Input: part model. Units: mm. Frame: model coordinates. Face numbers are marked on the shaded views. A direction names the side the tool comes from. Give positions to 0.01 mm unless a question says otherwise; leave off trailing zeros. Loops run counter-clockwise (first coordinate to the right, second up) from the corner with the lowest first, then second, coordinate; pieces in that order, holes last. Notation, with made-up numbers: M 31.25,14.25 L 56.25,14.25 A24 ccw 56.25,30.25 Z; hole C 75,46.25 d6. An arc over 180 degrees is marked long. Return JSON: item names as keys, results as strings. Group by question number.
```python
from build123d import *

# Parameters (mm, degrees)
EXTRUDE_1_DEPTH                 = 30
SKETCH_2_W                      = 3
SKETCH_2_H                      = 3
EXTRUDE_2_DEPTH                 = 1
EXTRUDE_START                   = -4
EXTRUDE_3_DEPTH                 = 5
CUT_EXTRUDE_1_REACH             = 52.312
CUT_EXTRUDE_1_DIRECTION_2_REACH = 52.312
FILLET_1_R                      = 0.1
PATTERN_LINEAR_1_COUNT          = 2
PATTERN_LINEAR_1_PITCH          = 15
PATTERN_LINEAR_1_COUNT_DIR2     = 2
PATTERN_LINEAR_1_PITCH_DIR2     = 15
FILLET_1_OF_PATTERN_LINEAR_1_R  = 0.1
FILLET_2_R                      = 0.2


with BuildPart() as part:
    # Sketch 1 → Extrude 1 (new body)
    with BuildSketch(Plane.XY):
        Polygon((-25.328427125, 0), (25.328427125, 0), (37.5, 12.171572875), (37.5, 15), (23.98, 2), (-23.98, 2), (-37.5, 15), (-37.5, 12.171572875), align=None)
    extrude(amount=-EXTRUDE_1_DEPTH)

    # Sketch 2 → Extrude 2 (add)
    with BuildSketch(Plane(origin=(0, 2, 0), x_dir=(1, 0, 0), z_dir=(0, 1, 0))):
        with Locations((0, 7.5)):
            Rectangle(SKETCH_2_W, SKETCH_2_H)
    extrude_2 = extrude(amount=EXTRUDE_2_DEPTH)

    # Sketch 3 → Extrude 3 (add)
    with BuildSketch(Plane.XY.offset(-6).offset(EXTRUDE_START)):
        with BuildLine():
            Line((-1.95, 4.5), (1.95, 4.5))
            Line((1.95, 4.5), (1.95, 3.555590279))
            ThreePointArc((1.95, 3.555590279), (1.780042303, 3.088161527), (1.5, 2.677124344))
            Line((1.5, 2.677124344), (-1.5, 2.677124344))
            ThreePointArc((-1.5, 2.677124344), (-1.780042303, 3.088161527), (-1.95, 3.555590279))
            Line((-1.95, 3.555590279), (-1.95, 4.5))
        make_face()
    extrude_3 = extrude(amount=EXTRUDE_3_DEPTH)

    # Sketch 4 → Cut-Extrude 1 (cut, up to next)
    with BuildSketch(Plane(origin=(0, 0, 0), x_dir=(0, 0, -1), z_dir=(1, 0, 0)), mode=Mode.PRIVATE) as cut_extrude_1_sk1:
        with BuildLine():
            Line((10, 4.5), (9.45, 4.5))
            Line((9.45, 4.5), (9.45, 3.555590279))
            ThreePointArc((9.45, 3.555590279), (9.280042303, 3.088161527), (9, 2.677124344))
            Line((9, 2.677124344), (10, 2.677124344))
            Line((10, 2.677124344), (10, 4.5))
        make_face()
    cut_extrude_1_tool1 = extrude(cut_extrude_1_sk1.sketch, amount=-CUT_EXTRUDE_1_REACH, mode=Mode.PRIVATE) & part.part
    # Sketch 4 → Cut-Extrude 1 (cut, up to next)
    with BuildSketch(Plane(origin=(0, 0, 0), x_dir=(0, 0, -1), z_dir=(1, 0, 0)), mode=Mode.PRIVATE) as cut_extrude_1_sk2:
        with BuildLine():
            Line((5, 4.5), (5, 2.677124344))
            Line((5, 2.677124344), (6, 2.677124344))
            ThreePointArc((6, 2.677124344), (5.719957697, 3.088161527), (5.55, 3.555590279))
            Line((5.55, 3.555590279), (5.55, 4.5))
            Line((5.55, 4.5), (5, 4.5))
        make_face()
    cut_extrude_1_tool2 = extrude(cut_extrude_1_sk2.sketch, amount=-CUT_EXTRUDE_1_REACH, mode=Mode.PRIVATE) & part.part
    cut_extrude_1_1 = cut_extrude_1_tool1.solids().sort_by_distance((0, 3.500125, -9.669375))[0]
    add(cut_extrude_1_1, mode=Mode.SUBTRACT)
    cut_extrude_1_2 = cut_extrude_1_tool2.solids().sort_by_distance((0, 3.500125, -5.330625))[0]
    add(cut_extrude_1_2, mode=Mode.SUBTRACT)
    cut_extrude_1 = cut_extrude_1_1 + cut_extrude_1_2  # Cut-Extrude 1 as one shape, for the pattern or mirror that repeats it

    # Sketch 4 → Cut-Extrude 1 direction 2 (cut, up to next)
    with BuildSketch(Plane(origin=(0, 0, 0), x_dir=(0, 0, -1), z_dir=(1, 0, 0)), mode=Mode.PRIVATE) as cut_extrude_1_direction_2_sk1:
        with BuildLine():
            Line((10, 4.5), (9.45, 4.5))
            Line((9.45, 4.5), (9.45, 3.555590279))
            ThreePointArc((9.45, 3.555590279), (9.280042303, 3.088161527), (9, 2.677124344))
            Line((9, 2.677124344), (10, 2.677124344))
            Line((10, 2.677124344), (10, 4.5))
        make_face()
    cut_extrude_1_direction_2_tool1 = extrude(cut_extrude_1_direction_2_sk1.sketch, amount=CUT_EXTRUDE_1_DIRECTION_2_REACH, mode=Mode.PRIVATE) & part.part
    # Sketch 4 → Cut-Extrude 1 direction 2 (cut, up to next)
    with BuildSketch(Plane(origin=(0, 0, 0), x_dir=(0, 0, -1), z_dir=(1, 0, 0)), mode=Mode.PRIVATE) as cut_extrude_1_direction_2_sk2:
        with BuildLine():
            Line((5, 4.5), (5, 2.677124344))
            Line((5, 2.677124344), (6, 2.677124344))
            ThreePointArc((6, 2.677124344), (5.719957697, 3.088161527), (5.55, 3.555590279))
            Line((5.55, 3.555590279), (5.55, 4.5))
            Line((5.55, 4.5), (5, 4.5))
        make_face()
    cut_extrude_1_direction_2_tool2 = extrude(cut_extrude_1_direction_2_sk2.sketch, amount=CUT_EXTRUDE_1_DIRECTION_2_REACH, mode=Mode.PRIVATE) & part.part
    cut_extrude_1_direction_2_1 = cut_extrude_1_direction_2_tool1.solids().sort_by_distance((0, 3.500125, -9.669375))[0]
    add(cut_extrude_1_direction_2_1, mode=Mode.SUBTRACT)
    cut_extrude_1_direction_2_2 = cut_extrude_1_direction_2_tool2.solids().sort_by_distance((0, 3.500125, -5.330625))[0]
    add(cut_extrude_1_direction_2_2, mode=Mode.SUBTRACT)
    cut_extrude_1_direction_2 = cut_extrude_1_direction_2_1 + cut_extrude_1_direction_2_2  # Cut-Extrude 1 direction 2 as one shape, for the pattern or mirror that repeats it

    # Fillet 1
    fillet_1_edges = [part.edges().sort_by_distance(p)[0] for p in [
        (1.95, 4.5, -7.5),
        (-1.95, 4.5, -7.5),
        (0, 4.5, -9.45),
        (0, 4.5, -5.55),
    ]]
    fillet(fillet_1_edges, radius=FILLET_1_R)

    # Pattern Linear 1: Extrude 2, Extrude 3, Cut-Extrude 1, Cut-Extrude 1 direction 2 2 × 2
    with Locations(*[Vector(1, 0, 0) * (i * PATTERN_LINEAR_1_PITCH) + Vector(-1, 0, 0) * (j * PATTERN_LINEAR_1_PITCH_DIR2) for i in range(PATTERN_LINEAR_1_COUNT) for j in range(PATTERN_LINEAR_1_COUNT_DIR2) if (i, j) != (0, 0)]):
        add(extrude_2)
        add(extrude_3)
        add(cut_extrude_1, mode=Mode.SUBTRACT)
        add(cut_extrude_1_direction_2, mode=Mode.SUBTRACT)

    # Fillet 1 of Pattern Linear 1
    fillet_1_of_pattern_linear_1_edges = [part.edges().sort_by_distance(p)[0] for p in [
        (-13.05, 4.5, -7.5),
        (-16.95, 4.5, -7.5),
        (-15, 4.5, -9.45),
        (-15, 4.5, -5.55),
        (16.95, 4.5, -7.5),
        (13.05, 4.5, -7.5),
        (15, 4.5, -9.45),
        (15, 4.5, -5.55),
        (1.95, 4.5, -7.5),
        (-1.95, 4.5, -7.5),
        (0, 4.5, -9.45),
        (0, 4.5, -5.55),
    ]]
    fillet(fillet_1_of_pattern_linear_1_edges, radius=FILLET_1_OF_PATTERN_LINEAR_1_R)

    # Fillet 2
    fillet_2_edges = [part.edges().sort_by_distance(p)[0] for p in [
        (0, 0, -30),
        (-31.414213562, 6.085786438, 0),
        (-37.5, 13.585786438, 0),
        (31.414213562, 6.085786438, -30),
        (-37.5, 15, -15),
        (37.5, 15, -15),
        (25.328427125, 0, -15),
        (-25.328427125, 0, -15),
        (37.5, 13.585786438, -30),
        (30.74, 8.5, -30),
        (0, 2, -30),
        (-30.74, 8.5, -30),
        (-37.5, 13.585786438, -30),
        (-31.414213562, 6.085786438, -30),
        (-30.74, 8.5, 0),
        (0, 2, 0),
        (30.74, 8.5, 0),
        (37.5, 13.585786438, 0),
        (31.414213562, 6.085786438, 0),
        (0, 0, 0),
    ]]
    fillet(fillet_2_edges, radius=FILLET_2_R)


solid = part.part
```
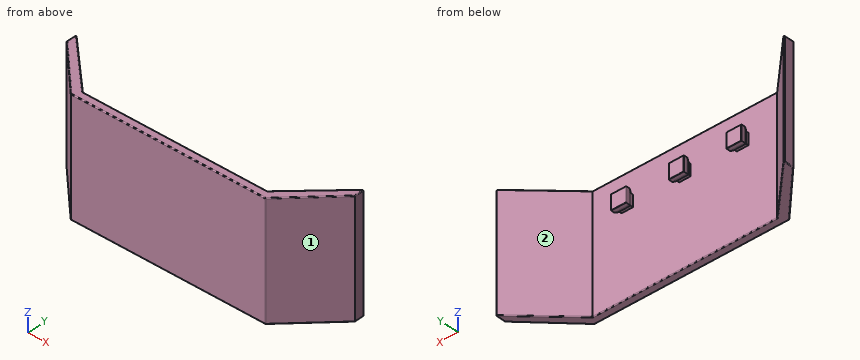
Item 1: Section B-B, the plane x = 4.5. Return loops of the section in (y, z), then the cut area to 3 significant figures.
Item 2: Section A-A, the plane z = -3.25. Return loops of the section in (x, y).
Item 3: First-contact query: pin 1 Ø0.7 at (y, z) = (4, -8) entering from -X; pin 2 Ø10 at (x, z) = (-24.5, -22.5) entering from +Y; pin 3 Ø0.5 at (y, z) = (2, -7) entering from +X. Flat tips, straight axial feed; report the tip coordinate or a pass-through.
Item 4: Reachability of the marked faces 1 and 2 from +Z, -Z, +X, -X, +Y, -Y: full face, straight path, thin tool, end or side. Return the list, or none.
Item 5: Material intervals for line 1 (X direction, y = 8.5, z = -21.75); line 2 (X direction, y = 11.5, z = -25.75); line 3 (Y direction, x = 11.5, z = -13.25), sorted ascending. Write a range as from..to.
Answer below:
{
 "1": {"outline": "M 0,-29.8 A0.2 ccw 0.2,-30 L 1.8,-30 A0.2 ccw 2,-29.8 L 2,-0.2 A0.2 ccw 1.8,0 L 0.2,0 A0.2 ccw 0,-0.2 Z", "area": "60.0 mm^2"},
 "2": {"outline": "M -37.5,12.17 L -25.39,0.06 A0.2 ccw -25.25,0 L 25.25,0 A0.2 ccw 25.39,0.06 L 37.5,12.17 L 37.5,14.53 A0.2 ccw 37.16,14.67 L 23.98,2 L -23.98,2 L -37.16,14.67 A0.2 ccw -37.5,14.53 Z"},
 "3": {"pin 1": "x = -29.68", "pin 2": "y = 7.31", "pin 3": "x = 27.58"},
 "4": {"face 1": "+Z, -Z, +X, -Y", "face 2": "+Z, -Z, +Y"},
 "5": {"line 1": "-33.83..-30.74, 30.74..33.83", "line 2": "-36.83..-33.86, 33.86..36.83", "line 3": "0..2"}
}
